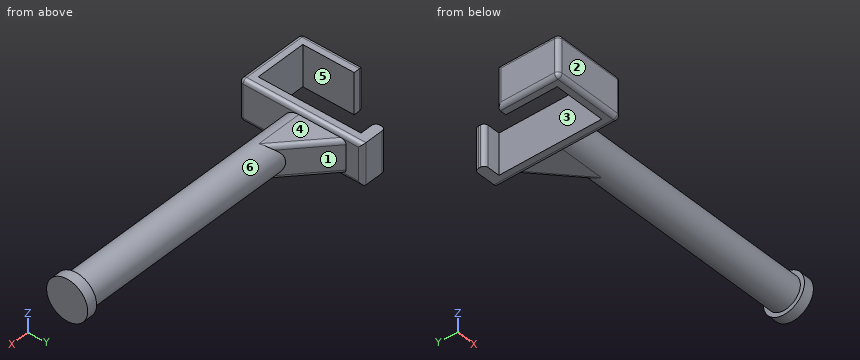
```python
from build123d import *

# Parameters (mm, degrees)
F1_DEPTH     = 10
F2_R         = 8
F3_DEPTH     = 125
F4_R         = 10
F4_R_2       = 8
F5_DEPTH     = 5
F7_DEPTH     = 8
F8_T4_DEPTH  = 47.7749887628
F8_S5_R      = 8
F8_T6_DEPTH  = 26
F8_T11_DEPTH = 47.7749887628
F8_S12_R     = 8
F8_T13_DEPTH = 26
F9_R         = 1.99999


# Not quite as in the source:
# - a fillet or chamfer that OpenCascade refuses, or shapes differently, is made with other operations: its cross-section is extruded or revolved along the edge and cut away or added
# - a fillet or chamfer is up to 0.001 mm smaller than in the source, because OpenCascade refuses the exact size


with BuildPart() as f1:
    # F0 (on Top) → F1 (new body, symmetric)
    with BuildSketch(Plane.XY):
        Polygon((-33.2763881331, -24.0594327205), (-33.2763881331, 0.9405672795), (-38.2763881331, 0.9405672795), (-38.2763881331, -29.0594327205), (-3.2763881331, -29.0594327205), (-3.2763881331, 30.9405672795), (-16.2763881331, 30.9405672795), (-16.2763881331, 25.9405672795), (-8.2763881331, 25.9405672795), (-8.2763881331, -24.0594327205), align=None)
    extrude(amount=F1_DEPTH, both=True)

    # F2 (on face) → F3 (join)
    with BuildSketch(Plane.YZ.offset(-3.2763881331)):
        Circle(F2_R)
    extrude(amount=F3_DEPTH)

    # F4 (on face) → F5 (join)
    with BuildSketch(Plane.YZ.offset(121.7236118669)):
        Circle(F4_R)
        Circle(F4_R_2, mode=Mode.SUBTRACT)
        Circle(F4_R_2)
    extrude(amount=F5_DEPTH)

    # F6 (on Top) → F7 (join, symmetric)
    with BuildSketch(Plane.XY):
        Polygon((22.1584475915, 0), (-4.7209444456, 24.2796987295), (-7.46962009, 0), align=None)
    extrude(amount=F7_DEPTH, both=True)

    # F8: fillet of radius 2 on 2 edges, made by hand


with BuildPart() as f8_tool2:
    # F8_s3 → F8_t4 (new body)
    with BuildSketch(Plane(origin=(18.5100171986, -16.719784452, 0), x_dir=(0, 0, 1), z_dir=(-0.742081519, 0.6703096442, 0))):
        with BuildLine():
            ThreePointArc((6, 14.8530211221), (7.4142135624, 14.2672346845), (8, 12.8530211221))
            Line((8, 12.8530211221), (8, 14.8530211221))
            Line((8, 14.8530211221), (6, 14.8530211221))
        make_face()
    extrude(amount=F8_T4_DEPTH)

    # F8_s5 → F8_t6 (cut, symmetric)
    with BuildSketch(Plane.YZ.offset(10.1)):
        Circle(F8_S5_R)
    extrude(amount=F8_T6_DEPTH, both=True, mode=Mode.SUBTRACT)

    split(bisect_by=Plane.YZ.offset(-3.2763881331), keep=Keep.TOP)


with BuildPart() as f1_1:
    add(f1.part)

    # F8_t1: cut F8_tool2
    add(f8_tool2.part, mode=Mode.SUBTRACT)


with BuildPart() as f8_tool9:
    # F8_s10 → F8_t11 (new body)
    with BuildSketch(Plane(origin=(18.5100171986, -16.719784452, 0), x_dir=(0, 0, 1), z_dir=(-0.742081519, 0.6703096442, 0))):
        with BuildLine():
            ThreePointArc((-6, 14.8530211221), (-7.4142135624, 14.2672346845), (-8, 12.8530211221))
            Line((-8, 12.8530211221), (-8, 14.8530211221))
            Line((-8, 14.8530211221), (-6, 14.8530211221))
        make_face()
    extrude(amount=F8_T11_DEPTH)

    # F8_s12 → F8_t13 (cut, symmetric)
    with BuildSketch(Plane.YZ.offset(10.1)):
        Circle(F8_S12_R)
    extrude(amount=F8_T13_DEPTH, both=True, mode=Mode.SUBTRACT)

    split(bisect_by=Plane.YZ.offset(-3.2763881331), keep=Keep.TOP)


with BuildPart() as f1_2:
    add(f1_1.part)

    # F8_t8: cut F8_tool9
    add(f8_tool9.part, mode=Mode.SUBTRACT)

    # F9 (radius 2 in the source; OpenCascade refuses exactly that, so slightly less here)
    f9_edges = [f1_2.edges().sort_by_distance(p)[0] for p in [
        (-3.276388, 0.940567, 10),
        (-3.276388, 0.940567, -10),
        (-20.776388, -29.059433, 10),
        (-20.776388, -29.059433, -10),
        (-38.276388, -14.059433, 10),
        (-38.276388, -14.059433, -10),
        (-38.276388, -29.059433, 0),
        (-38.276388, 0.940567, 0),
        (-3.276388, -29.059433, 0),
        (-3.276388, 30.940567, 0),
        (-16.276388, 30.940567, 0),
        (-16.276388, 25.940567, 0),
    ]]
    fillet(f9_edges, radius=F9_R)


solid = f1_2.part
```
Could you check a few things on this model? Use its own coordinates, in mm. Face numbers are marked on the shaded views. A direction names the side the tool comes from. Coordinates: 2 decimals unless noted, no trailing zeros. Loops run counter-clockwise (first coordinate to the right, second up) from the corner with the lowest first, then second, coordinate; pieces in that order, holes last. Notation, with made-up numbers: M -34,52.25 L 5,52.25 A17 cw 5,67.25 Z; hole C 27,17 d5. An arc over 180 degrees is marked long. Put each result on its own line as item: value. Start each with the question number.
(1) Will these pins go through, and if not, where does the flat tip stop? P1, Ø16, axis at x = 9.5, y = 10, coming from the +Z side; P2, Ø6, axis at x = 35, y = -8.5, coming from the -Z side; P3, Ø10, axis at x = 5, y = 5.5, coming from the -Z side.
(2) Suppose I cut it at A-A on y = -22.5. Please give me the cut outline in (x, z).
(3) Suppose I cut it at B-B on z = -2.75. Please give me the cut outline in (x, y).
(4) For the marked faces 4, 5 and 6, which set-ups out of +Z, -Z, +X, -X, +Y, -Y let a thin tool reach every point of the face, with its end or its side?
(5) Suppose I cut it at D-D on z = 4.5. Please give me the cut outline in (x, y), then the cut area to 3 significant figures.
(6) Thinking about a two-plate mould opening in Y: for the marked faces 1, 2 and 3, which applies, pulls with the +Y half, pulls with the -Y half, needs draft (parallel to the pull), parting line crosses it, or undercut?
(7) Suppose I cut it at C-C on x = 112. Please give me the cut outline in (y, z), then the cut area to 3 significant figures.
(8) I need wall thicknesses on line 1 (X direction, y = -8, z = -1); line 2 (X direction, y = -16.5, z = 6); line 3 (X direction, y = -5.5, z = 2.75). Which ranges of each line are inside material? Lowest first, please. Write a range as from..to.
Solutions:
1. P1: stops at z = 8
1. P2: stops at z = -5.81
1. P3: stops at z = -8
2. outline: M -38.28,-8 A2 ccw -36.28,-10 L -33.28,-10 L -33.28,10 L -36.28,10 A2 ccw -38.28,8 Z; M -8.28,-10 L -5.28,-10 A2 ccw -3.28,-8 L -3.28,8 A2 ccw -5.28,10 L -8.28,10 Z
3. outline: M -38.28,-27.06 A2 ccw -36.28,-29.06 L -5.28,-29.06 A2 ccw -3.28,-27.06 L -3.28,-7.51 L 121.72,-7.51 L 121.72,-9.61 L 126.72,-9.61 L 126.72,9.61 L 121.72,9.61 L 121.72,7.51 L 13.84,7.51 L -3.28,22.97 L -3.28,28.94 A2 ccw -5.28,30.94 L -14.28,30.94 A2 ccw -16.28,28.94 L -16.28,27.94 A2 ccw -14.28,25.94 L -8.28,25.94 L -8.28,-24.06 L -33.28,-24.06 L -33.28,0.94 L -36.28,0.94 A2 ccw -38.28,-1.06 Z
4. face 4: +Z, +Y, -Y
4. face 5: +Z, -Z, +Y
4. face 6: none
5. outline: M -38.28,-27.06 A2 ccw -36.28,-29.06 L -5.28,-29.06 A2 ccw -3.28,-27.06 L -3.28,-6.61 L 121.72,-6.61 L 121.72,-8.93 L 126.72,-8.93 L 126.72,8.93 L 121.72,8.93 L 121.72,6.61 L 14.84,6.61 L -3.28,22.97 L -3.28,28.94 A2 ccw -5.28,30.94 L -14.28,30.94 A2 ccw -16.28,28.94 L -16.28,27.94 A2 ccw -14.28,25.94 L -8.28,25.94 L -8.28,-24.06 L -33.28,-24.06 L -33.28,0.94 L -36.28,0.94 A2 ccw -38.28,-1.06 Z
5. area: 2,500 mm2
6. face 1: pulls with the +Y half
6. face 2: pulls with the -Y half
6. face 3: undercut
7. outline: C 0,0 d16
7. area: 201 mm2
8. line 1: x = -38.28..-33.28, -8.28..-3.28, 121.72..126.72
8. line 2: x = -38.28..-33.28, -8.28..-3.28
8. line 3: x = -38.28..-33.28, -8.28..126.72
